Build history of the part. All positions in model axes, mm. A direction names the side the tool comes from. Give positions to 0.01 mm unless a question says otherwise; leave off trailing zeros. Loops run counter-clockwise (first coordinate to the right, second up) from the corner with the lowest first, then second, coordinate; pieces in that order, holes last. Notation, with made-up numbers: M -11,30.25 L 9,30.25 A30 ccw 9,68.25 Z; hole C -27.75,23.5 d9. An arc over 180 degrees is marked long. Put each result on its own line as item: value.
```python
from build123d import *

# Parameters (mm, degrees)
SKETCH1_R           = 3.175
BOSS_EXTRUDE1_DEPTH = 3.175
SKETCH2_W           = 63.5
SKETCH2_H           = 2.54
EXTRUDE_THIN1_DEPTH = 25.4
SKETCH3_R           = 3.175
CUT_EXTRUDE1_DEPTH  = 25.4


with BuildPart() as part:
    # Sketch1 → Boss-Extrude1 (new body)
    with BuildSketch(Plane.XY):
        with BuildLine():
            Line((0, 0), (63.5, 0))
            Line((63.5, 0), (63.5, 15.875))
            Line((63.5, 15.875), (15.080341671, 64.294658329))
            ThreePointArc((15.080341671, 64.294658329), (8.505408108, 64.65221549), (11.339511683, 70.595737627))
            ThreePointArc((11.339511683, 70.595737627), (12.906539417, 71.462906002), (13.511840983, 73.148482141))
            ThreePointArc((13.511840983, 73.148482141), (8.586326617, 80.377738088), (0, 78.705067014))
            Line((0, 78.705067014), (0, 0))
        make_face()
        with Locations((9.525, 22.225)):
            Circle(SKETCH1_R, mode=Mode.SUBTRACT)
        with Locations((9.525, 53.975)):
            Circle(SKETCH1_R, mode=Mode.SUBTRACT)
        with Locations((41.275, 22.225)):
            Circle(SKETCH1_R, mode=Mode.SUBTRACT)
    extrude(amount=BOSS_EXTRUDE1_DEPTH)

    # Sketch2 → Extrude-Thin1 (add)
    with BuildSketch(Plane(origin=(0, 0, 0), x_dir=(-1, 0, 0), z_dir=(0, 0, -1))):
        with Locations((-31.75, 1.905)):
            Rectangle(SKETCH2_W, SKETCH2_H)
    extrude(amount=EXTRUDE_THIN1_DEPTH)

    # Sketch3 → Cut-Extrude1 (cut)
    with BuildSketch(Plane(origin=(0, 3.175, 0), x_dir=(1, 0, 0), z_dir=(0, 1, 0))):
        with Locations(Location((31.75, 12.7, 0), (0, 0, 180))):
            Circle(SKETCH3_R)
        with Locations(Location((9.525, 15.875, 0), (0, 0, 180))):
            Circle(SKETCH3_R)
        with Locations(Location((56.699380445, 15.875, 0), (0, 0, 180))):
            Circle(SKETCH3_R)
    extrude(amount=-CUT_EXTRUDE1_DEPTH, mode=Mode.SUBTRACT)


solid = part.part
```
Q1. Tool access for faces 4 (the flat face through (32, 3.175, -7)), 5 (the cylindrical face through (12.697, 1.923, -15.735)), 6 (the cylindrical face through (12.89, 71.443, 1.565)): list every direction of +Z, -Z, +X, -X, +Y, -Y with a clear straight run to the whole face (end or side of a thin tool).
Here are the results:
face 4: -Z, +X, -X, +Y
face 5: +Y, -Y
face 6: +Z, -Z, +X
Q2. Slice it at C-C (y = 13.5). List the corners of the cut face in (x, z) (3 decimals).
Here are the results:
outline: M 0,0 L 63.5,0 L 63.5,3.175 L 0,3.175 Z
Q3. Slice it at D-D (x = 5). List the corners of the cut face in (y, z) (3 decimals), and give its area (3 significant figures).
Here are the results:
outline: M 0,0 L 0.635,0 L 0.635,-25.4 L 3.175,-25.4 L 3.175,0 L 80.955,0 L 80.955,3.175 L 0,3.175 Z
area: 322 mm²
Q4. Drop flat-ended pins along their axis: pin 1 Ø7.5 at (x, z) = (9.525, -15.875) entering from +Y (3 decimals); pin 2 Ø10 at (y, z) = (40, -9) entering from +X; pin 3 Ø6 at (x, z) = (46, -18.5) entering from -Y (3 decimals); pin 4 Ø1.5 at (x, y) = (39, 29.5) entering from -Z. Give the stop position or say it passes through.
Here are the results:
pin 1: y = 3.175
pin 2: through
pin 3: y = 0.635
pin 4: z = 0
Q5. Slice it at B-B (z = -1.25). List the corners of the cut face in (x, y) (3 decimals).
Here are the results:
outline: M 0,0.635 L 63.5,0.635 L 63.5,3.175 L 0,3.175 Z
Q6. Mould opens along Y. For faces 1 (the cylindrical face through (8.56, 64.56, 1.57)), 2 (the cylindrical face through (8.706, 80.327, 1.565)), 3 (the flat face through (32, 0.635, -7)) say: pulls with the +Y half, pulls with the -Y half, needs draft (parallel to the pull), parting line crosses it, or undercut.
Here are the results:
face 1: undercut
face 2: pulls with the +Y half
face 3: pulls with the -Y half
Q7. Slice it at A-A (x = 31.75). List the corners of the cut face in (y, z) (3 decimals).
Here are the results:
outline: M 0,0 L 0.635,0 L 0.635,-9.525 L 3.175,-9.525 L 3.175,0 L 47.625,0 L 47.625,3.175 L 0,3.175 Z; M 0.635,-25.4 L 3.175,-25.4 L 3.175,-15.875 L 0.635,-15.875 Z
Q8. Probe line 1 (Y direction, x = 42, z = -9.5) (3 decimals); line 2 (Z direction, x = 11, y = 8) (3 decimals); line 3 (X direction, y = 30, z = 1.75) (3 decimals). List the from-to ranges inside material, lowest first. Write a range as from..to.
Here are the results:
line 1: 0.635..3.175
line 2: 0..3.175
line 3: 0..49.375
